Check sheet for the modelled part. Datum: model origin and axes. Units: mm. Face numbers are marked on the shaded views. A direction names the side the tool comes from. Round coordinates to 2 decimals unless told otherwise and drop trailing zeros. Order: outer loops, then holes, each group sorted by start corner. A loop starts at its lowest first (then second) coordinate and runs counter-clockwise, first axis right, second up.
(1) Tool access check on the marked faces 1 and 2. Record the directions out of +Z, -Z, +X, -X, +Y, -Y that give a thin tool (end or side, any length) a straight path to the whole face; none if there is none.
(2) Depth check by flat-ended pin: pin 1 (3 mm diameter, centred on x = 0, z = 0, fed in from +Y); pin 2 (1.5 mm diameter, centred on x = -2.5, y = -5.5, fed in from -Z); pin 3 (2 mm diameter, centred on x = -2.5, y = -7, fed in from +Z). Enter the tip coordinate at first touch or a pass-through.
(3) Sectioned sample at D-D, the plane y = -8.25. Enter the section's corners in (x, z), and give its area (3 significant figures).
(4) Sectioned sample at B-B, the plane z = 0. Enter the section's corners in (x, y).
(5) Sectioned sample at C-C, the plane y = -2.5. Enter the section's corners in (x, z), and give its area (3 significant figures).
(6) Thickness scan on probe 1 along Y at (x, z) = (0.5, 0.5); probe 2 along X at (y, z) = (-2.5, 0.75); probe 3 along Z at (x, y) = (-1, -2.75). Record the ranges inside material, lowest first.
(7) Mould release check, pull along Z, two halves, no side actions. Record for the marked faces 3, 4 and 5: released by +Z, released by -Z, zero draft, split by the parting line, or undercut.
(8) Sectioned sample at A-A, the plane x = 0. Enter the section's corners in (y, z).
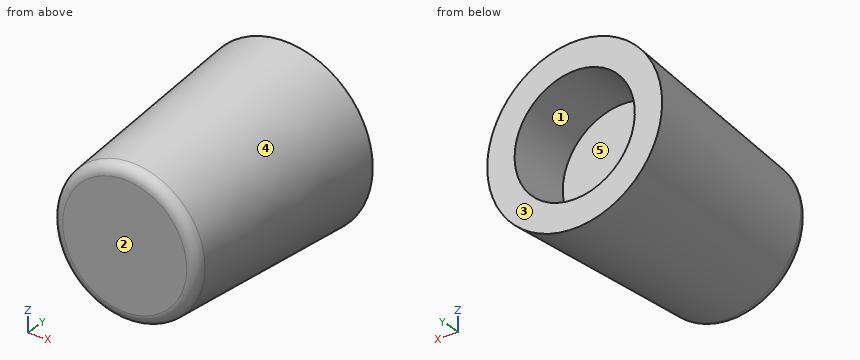
```python
from build123d import *

# Parameters (mm, degrees)
SKETCH1_R               = 4
BOSS_EXTRUDE1_DEPTH     = 10
BOSS_EXTRUDE1_DRAFT     = -4
SKETCH2_R               = 2.75
BOSS_EXTRUDE2_DEPTH     = 3
CUT_EXTRUDE1_DEPTH      = 12.489125293
CUT_EXTRUDE1_DEPTH_BACK = 3
SKETCH2_3_R             = 2.75
FILLET1_R               = 0.5


with BuildPart() as part:
    # Sketch1 → Boss-Extrude1 (with draft: the straight prism first)
    with BuildSketch(Plane(origin=(0, 0, 0), x_dir=(1, 0, 0), z_dir=(0, 1, 0))):
        Circle(SKETCH1_R)
    extrude(amount=-BOSS_EXTRUDE1_DEPTH)
    # Boss-Extrude1: the draft: its side faces are tilted about the plane it starts from
    boss_extrude1_sides = [part.faces().sort_by_distance(p)[0] for p in [
        (-4, -5, 0),
    ]]
    draft(boss_extrude1_sides, Plane(origin=(0, 0, 0), x_dir=(1, 0, 0), z_dir=(0, 1, 0)), BOSS_EXTRUDE1_DRAFT)

    # Sketch2 → Boss-Extrude2 (add)
    with BuildSketch(Plane(origin=(0, 0, 0), x_dir=(1, 0, 0), z_dir=(0, 1, 0))):
        Circle(SKETCH2_R)
    extrude(amount=-BOSS_EXTRUDE2_DEPTH)

    # Sketch2_3 → Cut-Extrude1 (cut, two sides: drawn at the far end of the back side and taken through both)
    with BuildSketch(Plane(origin=(0, 0, 0), x_dir=(1, 0, 0), z_dir=(0, 1, 0)).offset(-CUT_EXTRUDE1_DEPTH_BACK)):
        with Locations(Location((0, 0, 0), (0, 0, 90))):
            Circle(SKETCH2_3_R)
    extrude(amount=CUT_EXTRUDE1_DEPTH + CUT_EXTRUDE1_DEPTH_BACK, mode=Mode.SUBTRACT)

    # Fillet1
    fillet1_edges = [part.edges().sort_by_distance(p)[0] for p in [
        (-3.300731881, -10, 0),
    ]]
    fillet(fillet1_edges, radius=FILLET1_R)


solid = part.part
```
Derived:
1. face 1: +Y
1. face 2: +Z, -Z, +X, -X, -Y
2. pin 1: stops at y = -3
2. pin 2: stops at z = -3.17
2. pin 3: stops at z = 3.18
3. outline: circle Ø6.85 at (0, 0)
3. area: 36.8 mm2
4. outline: (-4, 0) - (-3.33, -9.53) arc R0.5 ccw to (-2.83, -10) - (2.83, -10) arc R0.5 ccw to (3.33, -9.53) - (4, 0) - (2.75, 0) - (2.75, -3) - (-2.75, -3) - (-2.75, 0) - close
5. outline: circle Ø7.65 at (0, 0); hole circle Ø5.5 at (0, 0)
5. area: 22.2 mm2
6. probe 1: y = -10 to -3
6. probe 2: x = -3.75 to -2.65, 2.65 to 3.75
6. probe 3: z = -3.67 to -2.56, 2.56 to 3.67
7. face 3: zero draft
7. face 4: split by the parting line
7. face 5: undercut
8. outline: (-10, -2.83) arc R0.5 ccw to (-9.53, -3.33) - (0, -4) - (0, -2.75) - (-3, -2.75) - (-3, 2.75) - (0, 2.75) - (0, 4) - (-9.53, 3.33) arc R0.5 ccw to (-10, 2.83) - close
